The listing builds one solid part. Answer for the finished solid, in the listing's coordinates (mm). A direction names the side the tool comes from. Coordinates: 2 decimals unless noted, no trailing zeros. Loops run counter-clockwise (first coordinate to the right, second up) from the corner with the lowest first, then second, coordinate; pieces in that order, holes last. Notation, with made-up numbers: (71, -7.75) - (109, -7.75) arc R25 cw to (109, 4.25) - close; hole circle Ø10 at (75, 18). An arc over 180 degrees is marked (long way). Return JSON: item names as keys, results as strings. Group by question number.
1. Which of the six approach directions +Z, -Z, +X, -X, +Y, -Y give full straight-line access (tool end or side, diameter ignored) to faces 4 (the face through (135, 39, 15)), 5 (the face through (109, 30, 147)), 6 (the face through (146, 30, 109))?
2. Each of these flat-tipped pins is pushed along its axis until it touches: P1, Ø18, axis at x = 135, z = 134, coming from the +Y side; P2, Ø24, axis at x = 139, z = 139, coming from the +Y side; P3, Ø2, axis at y = 86.5, z = 113, coming from the -X side. Where does it stop, or does it pass through?
3. Section A-A (x = 139) is taken. Write down the section's boundary in (y, z).
4. Find the intervals of material crossed by line 1 along Z through (x, y) = (139, 31.25); line 2 along Z through (x, y) = (139, 8.5); line 3 along Y through (x, z) = (7, 146), in increasing order.
5. Section C-C (x = 164) is taken. Write down the section's boundary in (y, z), and give its area (3 significant figures).
6. Section D-D (x = 7.5) is taken. Write down the section's boundary in (y, z), and give its area (3 significant figures).
7. The mould has two halves that part along Y. Classify faces 1 (the face through (76.99, 14.86, -28.15)), 2 (the face through (135, 25, 132)), 3 (the face through (169, 15, 63)): pulls with the +Y half, pulls with the -Y half, needs draft (parallel to the pull), parting line crosses it, or undercut.
8. Section B-B (z = 139) is taken. Write down the section's boundary in (x, y), and give its area (3 significant figures).
```python
from build123d import *

# Parameters (mm, degrees)
BOSS_EXTRUDE1_DEPTH                     = 25
BOSS_EXTRUDE2_START                     = -25
BOSS_EXTRUDE2_DEPTH                     = 95
BOSS_EXTRUDE3_DEPTH                     = 10
CBORE_FOR_M8_HEX_HEAD_BOLT1_D           = 15
CBORE_FOR_M8_HEX_HEAD_BOLT1_CBORE_D     = 30
CBORE_FOR_M8_HEX_HEAD_BOLT1_CBORE_DEPTH = 10
CUT_EXTRUDE1_DEPTH                      = 20
BOSS_EXTRUDE4_START                     = 10
SKETCH7_R                               = 34.833333333
BOSS_EXTRUDE4_DEPTH                     = 125
BOSS_EXTRUDE5_START                     = 10
SKETCH8_R                               = 41.333333333
BOSS_EXTRUDE5_DEPTH                     = 125
CUT_EXTRUDE2_REACH                      = 315.988
SKETCH9_R                               = 20.5
CUT_EXTRUDE3_REACH                      = 322.331
SKETCH10_R                              = 20.5
CHAMFER1_SIZE                           = 2
CUT_EXTRUDE4_DEPTH                      = 20
FILLET1_R                               = 10


with BuildPart() as part:
    # Sketch1 → Boss-Extrude1 (new body)
    with BuildSketch(Plane(origin=(0, 0, 0), x_dir=(1, 0, 0), z_dir=(0, 1, 0))):
        with BuildLine():
            Line((-39, 40), (159, 40))
            ThreePointArc((159, 40), (166.071067812, 37.071067812), (169, 30))
            Line((169, 30), (169, -159))
            ThreePointArc((169, -159), (166.071067812, -166.071067812), (159, -169))
            Line((159, -169), (-39, -169))
            ThreePointArc((-39, -169), (-46.071067812, -166.071067812), (-49, -159))
            Line((-49, -159), (-49, 30))
            ThreePointArc((-49, 30), (-46.071067812, 37.071067812), (-39, 40))
        make_face()
    extrude(amount=BOSS_EXTRUDE1_DEPTH)

    # Sketch2 → Boss-Extrude2 (add)
    with BuildSketch(Plane(origin=(0, 25, 0), x_dir=(1, 0, 0), z_dir=(0, 1, 0)).offset(BOSS_EXTRUDE2_START)):
        with BuildLine():
            Line((0, -89), (0, -169))
            Line((0, -169), (15, -169))
            Line((15, -169), (15, -102.912584265))
            ThreePointArc((15, -102.912584265), (73.539105243, -73.539105243), (102.912584265, -15))
            Line((102.912584265, -15), (169, -15))
            Line((169, -15), (169, 0))
            Line((169, 0), (89, 0))
            ThreePointArc((89, 0), (62.932503526, -62.932503526), (0, -89))
        make_face()
    extrude(amount=BOSS_EXTRUDE2_DEPTH)

    # Sketch3 → Boss-Extrude3 (add)
    with BuildSketch(Plane(origin=(0, 25, 0), x_dir=(1, 0, 0), z_dir=(0, 1, 0))):
        with BuildLine():
            Line((124, -109), (169, -109))
            Line((169, -109), (169, -159))
            ThreePointArc((169, -159), (166.071067812, -166.071067812), (159, -169))
            Line((159, -169), (109, -169))
            Line((109, -169), (109, -124))
            ThreePointArc((109, -124), (113.393398282, -113.393398282), (124, -109))
        make_face()
    extrude(amount=BOSS_EXTRUDE3_DEPTH)

    # CBORE for M8 Hex Head Bolt1 (through all)
    with Locations(Plane(origin=(0, 35, 0), x_dir=(1, 0, 0), z_dir=(0, 1, 0))):
        with Locations((139, -139)):
            CounterBoreHole(CBORE_FOR_M8_HEX_HEAD_BOLT1_D / 2, CBORE_FOR_M8_HEX_HEAD_BOLT1_CBORE_D / 2, CBORE_FOR_M8_HEX_HEAD_BOLT1_CBORE_DEPTH)

    # Sketch6 → Cut-Extrude1 (cut)
    with BuildSketch(Plane(origin=(0, 25, 0), x_dir=(1, 0, 0), z_dir=(0, 1, 0))):
        with BuildLine():
            Line((100, -150), (100, -124))
            ThreePointArc((100, -124), (107.029437252, -107.029437252), (124, -100))
            Line((124, -100), (150, -100))
            ThreePointArc((150, -100), (157.071067812, -97.071067812), (160, -90))
            Line((160, -90), (160, -34))
            ThreePointArc((160, -34), (157.071067812, -26.928932188), (150, -24))
            Line((150, -24), (118.207444774, -24))
            ThreePointArc((118.207444774, -24), (112.192558093, -26.011186683), (108.59708341, -31.235772358))
            ThreePointArc((108.59708341, -31.235772358), (79.903066274, -79.903066274), (31.235772358, -108.59708341))
            ThreePointArc((31.235772358, -108.59708341), (26.011186683, -112.192558093), (24, -118.207444774))
            Line((24, -118.207444774), (24, -150))
            ThreePointArc((24, -150), (26.928932188, -157.071067812), (34, -160))
            Line((34, -160), (90, -160))
            ThreePointArc((90, -160), (97.071067812, -157.071067812), (100, -150))
        make_face()
    extrude(amount=-CUT_EXTRUDE1_DEPTH, mode=Mode.SUBTRACT)

    # Sketch7 → Boss-Extrude4 (add)
    with BuildSketch(Plane.XY.offset(169).offset(BOSS_EXTRUDE4_START)):
        with Locations((7.5, 95)):
            Circle(SKETCH7_R)
    extrude(amount=-BOSS_EXTRUDE4_DEPTH)

    # Sketch8 → Boss-Extrude5 (add)
    with BuildSketch(Plane(origin=(169, 0, 0), x_dir=(0, 0, -1), z_dir=(1, 0, 0)).offset(BOSS_EXTRUDE5_START)):
        with Locations((-7.5, 95)):
            Circle(SKETCH8_R)
    extrude(amount=-BOSS_EXTRUDE5_DEPTH)

    # Sketch9 → Cut-Extrude2 (cut, up to next)
    with BuildSketch(Plane.XY.offset(179), mode=Mode.PRIVATE) as cut_extrude2_sk1:
        with Locations((7.5, 95)):
            Circle(SKETCH9_R)
    cut_extrude2_tool1 = extrude(cut_extrude2_sk1.sketch, amount=-CUT_EXTRUDE2_REACH, mode=Mode.PRIVATE) & part.part
    add(cut_extrude2_tool1.solids().sort_by_distance((7.5, 95, 179))[0], mode=Mode.SUBTRACT)

    # Sketch10 → Cut-Extrude3 (cut, up to next)
    with BuildSketch(Plane(origin=(179, 0, 0), x_dir=(0, 0, -1), z_dir=(1, 0, 0)), mode=Mode.PRIVATE) as cut_extrude3_sk1:
        with Locations((-7.5, 95)):
            Circle(SKETCH10_R)
    cut_extrude3_tool1 = extrude(cut_extrude3_sk1.sketch, amount=-CUT_EXTRUDE3_REACH, mode=Mode.PRIVATE) & part.part
    add(cut_extrude3_tool1.solids().sort_by_distance((179, 95, 7.5))[0], mode=Mode.SUBTRACT)

    # Chamfer1
    chamfer1_edges = [part.edges().sort_by_distance(p)[0] for p in [
        (-13, 95, 179),
        (-13, 95, 54),
        (179, 95, 28),
        (54, 95, 28),
    ]]
    chamfer(chamfer1_edges, length=CHAMFER1_SIZE)

    # Sketch11 → Cut-Extrude4 (cut)
    with BuildSketch(Plane(origin=(0, 25, 0), x_dir=(1, 0, 0), z_dir=(0, 1, 0))):
        with BuildLine():
            Line((0, -80), (-40, -80))
            Line((-40, -80), (-40, 30))
            Line((-40, 30), (-40, 31))
            Line((-40, 31), (-39, 31))
            Line((-39, 31), (80, 31))
            Line((80, 31), (80, 0))
            ThreePointArc((80, 0), (56.568542495, -56.568542495), (0, -80))
        make_face()
    extrude(amount=-CUT_EXTRUDE4_DEPTH, mode=Mode.SUBTRACT)

    # Fillet1
    fillet1_edges = [part.edges().sort_by_distance(p)[0] for p in [
        (-40, 15, 80),
        (-40, 15, -31),
        (80, 15, -31),
    ]]
    fillet(fillet1_edges, radius=FILLET1_R)


solid = part.part
```
The answers:
{
 "1": {"face 4": "+X", "face 5": "+Z, +Y", "face 6": "+X, +Y"},
 "2": {"P1": "stops at y = 35", "P2": "stops at y = 25", "P3": "stops at x = -26.52"},
 "3": {"outline": "(0, -40) - (25, -40) - (25, 0) - (54.35, 0) arc R41.33 ccw (long way) to (54.35, 15) - (25, 15) - (25, 24) - (5, 24) - (5, 100) - (25, 100) - (25, 109) - (35, 109) - (35, 124) - (25, 124) - (25, 131.5) - (0, 131.5) - close; (0, 146.5) - (25, 146.5) - (25, 154) - (35, 154) - (35, 169) - (0, 169) - close; hole circle Ø41 at (95, 7.5)"},
 "4": {"line 1": "z = 0 to 15, 109 to 124, 154 to 169", "line 2": "z = -40 to 24, 100 to 131.5, 146.5 to 169", "line 3": "y = 0 to 74.51, 115.49 to 129.83"},
 "5": {"outline": "(0, -38.66) - (25, -38.66) - (25, 0) - (54.35, 0) arc R41.33 ccw (long way) to (54.35, 15) - (25, 15) - (25, 109) - (35, 109) - (35, 167.66) - (0, 167.66) - close; hole circle Ø41 at (95, 7.5)", "area": "10,200 mm2"},
 "6": {"outline": "(0, -40) - (25, -40) - (25, -31) - (5, -31) - (5, 79.65) - (25, 79.65) - (25, 88.68) - (60.17, 88.68) - (60.17, 54) - (72.5, 54) - (74.5, 56) - (74.5, 177) - (72.5, 179) - (60.17, 179) - (60.17, 169) - (0, 169) - close; (115.5, 56) - (117.5, 54) - (129.83, 54) - (129.83, 179) - (117.5, 179) - (115.5, 177) - close", "area": "9,410 mm2"},
 "7": {"face 1": "undercut", "face 2": "pulls with the +Y half", "face 3": "needs draft"},
 "8": {"outline": "(-49, 0) - (131.5, 0) - (131.5, 25) - (124, 25) - (124, 35) - (109, 35) - (109, 25) - (100, 25) - (100, 5) - (24, 5) - (24, 25) - (15, 25) - (15, 60.98) arc R34.83 ccw (long way) to (0, 60.98) - (0, 25) - (-49, 25) - close; (146.5, 0) - (169, 0) - (169, 35) - (154, 35) - (154, 25) - (146.5, 25) - close; hole circle Ø41 at (7.5, 95)", "area": "6,880 mm2"}
}
